CAD build for the part. Positions are in the model's coordinates, mm. A direction names the side the tool comes from. Round coordinates to 2 decimals unless told otherwise and drop trailing zeros. Order: outer loops, then holes, each group sorted by start corner. A loop starts at its lowest first (then second) coordinate and runs counter-clockwise, first axis right, second up. Notation, with made-up numbers: M 64.25,59.25 L 99.25,59.25 A27 cw 99.25,92.25 Z; hole C 86.25,17 d7. An arc over 180 degrees is marked long. Answer as a JSON object with one key per item and string values.
```python
from build123d import *

# Parameters (mm, degrees)
F0_W     = 5.08
F0_H     = 5.08
F1_DEPTH = 7.62
F2_W     = 5.08
F2_H     = 12.7
F3_DEPTH = 2.54
F4_R     = 2.53999


# Not quite as in the source:
# - a fillet or chamfer is up to 0.001 mm smaller than in the source, because OpenCascade refuses the exact size


with BuildPart() as f1:
    # F0 (on Front) → F1 (new body)
    with BuildSketch(Plane.XZ):
        Rectangle(F0_W, F0_H)
    extrude(amount=F1_DEPTH)

    # F2 (on face) → F3 (join)
    with BuildSketch(Plane.XZ.offset(7.62)):
        with Locations((0, -3.81)):
            Rectangle(F2_W, F2_H)
    extrude(amount=F3_DEPTH)

    # F4 (radius 2.54 in the source; OpenCascade refuses exactly that, so slightly less here)
    f4_edges = [f1.edges().sort_by_distance(p)[0] for p in [
        (0, -10.16, 2.54),
        (0, -10.16, -10.16),
    ]]
    fillet(f4_edges, radius=F4_R)


solid = f1.part
```
Item 1: Wall check: line 1 along Z through (x, y) = (-1.8, -6); line 2 along Y through (x, z) = (0.5, -7.5); line 3 along Z through (x, y) = (-1.4, -7.75). Give the ranges that are in metal, low to high. Write a range as [from, to].
Worked answers:
{"line 1": "z = [-2.54, 2.54]", "line 2": "y = [-10.16, -7.62]", "line 3": "z = [-10.16, 2.54]"}
Item 2: 3-axis set-ups, long thin cutter, end or side, ignore diameter. For faces 1 (the flat face through (0, -10.16, -4)), 2 (the flat face through (0, -4, -2.54)): which of +Z, -Z, +X, -X, +Y, -Y reach the whole face in a straight line?
Worked answers:
{"face 1": "+Z, -Z, +X, -X, -Y", "face 2": "-Z, +X, -X, +Y"}
Item 3: Saw through at B-B on y = -1.5. List the corners of the cut face in (x, z), and give its area (3 significant figures).
Worked answers:
{"outline": "M -2.54,-2.54 L 2.54,-2.54 L 2.54,2.54 L -2.54,2.54 Z", "area": "25.8 mm2"}
Item 4: Saw through at C-C on z = -5.5. List the corners of the cut face in (x, y), and give its area (3 significant figures).
Worked answers:
{"outline": "M -2.54,-10.16 L 2.54,-10.16 L 2.54,-7.62 L -2.54,-7.62 Z", "area": "12.9 mm2"}
Item 5: Drop flat-ended pins along their axis: pin 1 Ø1.5 at (x, z) = (-0.5, -7.5) entering from +Y; pin 2 Ø3 at (x, y) = (-0.5, -8) entering from +Z; pin 3 Ø1.5 at (x, y) = (-0.5, -2.5) entering from -Z. Give the stop position or say it passes through.
Worked answers:
{"pin 1": "stops at y = -7.62", "pin 2": "stops at z = 2.54", "pin 3": "stops at z = -2.54"}
